Input: part model. Units: mm. Frame: model coordinates. Face numbers are marked on the shaded views. A direction names the side the tool comes from. Round coordinates to 2 decimals unless told otherwise and drop trailing zeros. Loops run counter-clockwise (first coordinate to the right, second up) from the corner with the lowest first, then second, coordinate; pieces in that order, holes last.
1) Section D-D, the plane z = 12. Return loops of the section in (x, y).
2) Section B-B, the plane y = -20. Return loops of the section in (x, z), and give its area (3 significant figures).
3) Section C-C, the plane x = 20. Return loops of the section in (y, z), and give its area (3 significant figures).
4) First-contact query: pin 1 (1.5 mm diameter, centred on y = -16, z = -5.5, fed in from -X); pin 2 (12 mm diameter, centred on x = 0, z = 0, fed in from -Y); pin 3 (1 mm diameter, centred on y = 13, z = -7, fed in from +X); pin 4 (3 mm diameter, centred on x = 23, y = -5.5, fed in from -Z). Flat tips, straight axial feed; report the tip coordinate or a pass-through.
5) Access query for the marked faces 1, 2 and 3. Directions: +Z, -Z, +X, -X, +Y, -Y. A direction counts if a zero-diameter tool reaches every point of the face in a straight line with its end or side. Return the directions, or none.
6) Ray query, line 1 along Y through (x, z) = (-20, 1); line 2 along Y through (x, z) = (18.5, 2.5); line 3 along Z through (x, y) = (0, -11). Return the intervals inside material, ascending.
7) Draft query along X for the marked faces 4, 5, 6 and 7. Return one class per face: pulls with the +X half, pulls with the -X half, needs draft (parallel to the pull), parting line crosses it, or undercut.
8) Section A-A, the plane z = -6. Return loops of the section in (x, y).
from build123d import *

# Parameters (mm, degrees)
F0_R     = 10
F1_DEPTH = 25
F2_R     = 2
F3_DEPTH = 40


with BuildPart() as f1:
    # F0 (on Front) → F1 (new body, symmetric)
    with BuildSketch(Plane.XZ):
        Polygon((-15, -14), (-9.5, -20), (9.5, -20), (15, -14), (25.5, -14), (25.5, 9.815577), (27, 11.315577), (27, 19.5), (25.5, 21), (14.5, 21), (13, 19.5), (-13, 19.5), (-14.5, 21), (-25.5, 21), (-27, 19.5), (-27, 11.315577), (-25.5, 9.815577), (-25.5, -14), align=None)
        Circle(F0_R, mode=Mode.SUBTRACT)
    extrude(amount=F1_DEPTH, both=True)

    # F2 (on face) → F3 (cut)
    with BuildSketch(Plane.XY.offset(21)):
        with Locations((-20, 20)):
            Circle(F2_R)
        with Locations((20, 20)):
            Circle(F2_R)
        with Locations((20, -20)):
            Circle(F2_R)
        with Locations((-20, -20)):
            Circle(F2_R)
    extrude(amount=-F3_DEPTH, mode=Mode.SUBTRACT)


solid = f1.part
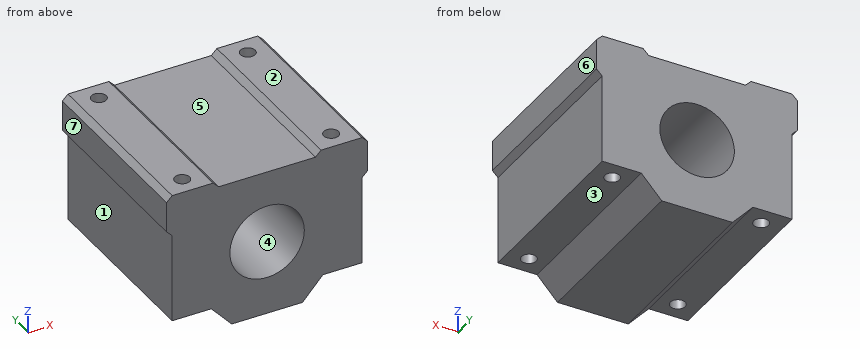
Final values:
1. outline: (-27, -25) - (27, -25) - (27, 25) - (-27, 25) - close; hole circle Ø4 at (-20, -20); hole circle Ø4 at (-20, 20); hole circle Ø4 at (20, -20); hole circle Ø4 at (20, 20)
2. outline: (-27, 11.32) - (-25.5, 9.82) - (-25.5, -14) - (-22, -14) - (-22, 21) - (-25.5, 21) - (-27, 19.5) - close; (-18, -14) - (-15, -14) - (-9.5, -20) - (9.5, -20) - (15, -14) - (18, -14) - (18, 21) - (14.5, 21) - (13, 19.5) - (-13, 19.5) - (-14.5, 21) - (-18, 21) - close; (22, -14) - (25.5, -14) - (25.5, 9.82) - (27, 11.32) - (27, 19.5) - (25.5, 21) - (22, 21) - close; hole circle Ø20 at (0, 0)
2. area: 1,330 mm2
3. outline: (-25, -14) - (-22, -14) - (-22, 21) - (-25, 21) - close; (-18, -14) - (18, -14) - (18, 21) - (-18, 21) - close; (22, -14) - (25, -14) - (25, 21) - (22, 21) - close
3. area: 1,470 mm2
4. pin 1: stops at x = -25.5
4. pin 2: passes through
4. pin 3: stops at x = 25.5
4. pin 4: stops at z = -14
5. face 1: -Z, -X, +Y, -Y
5. face 2: +Z, +X, -X, +Y, -Y
5. face 3: -Z, +X, +Y, -Y
6. line 1: y = -25 to -22, -18 to 18, 22 to 25
6. line 2: y = -25 to -21.32, -18.68 to 18.68, 21.32 to 25
6. line 3: z = -20 to -10, 10 to 19.5
7. face 4: undercut
7. face 5: undercut
7. face 6: pulls with the +X half
7. face 7: pulls with the -X half
8. outline: (-25.5, -25) - (-8, -25) - (-8, 25) - (-25.5, 25) - close; (8, -25) - (25.5, -25) - (25.5, 25) - (8, 25) - close; hole circle Ø4 at (-20, -20); hole circle Ø4 at (-20, 20); hole circle Ø4 at (20, -20); hole circle Ø4 at (20, 20)
